Autodesk Inventor part; units mm, degrees
ref_plane "YZ Plane" through (0, 0, 0) normal (1, 0, 0) x (0, 1, 0)
ref_plane "XZ Plane" through (0, 0, 0) normal (0, 1, 0) x (-1, 0, 0)
ref_plane "XY Plane" through (0, 0, 0) normal (0, 0, 1) x (1, 0, 0)
sketch "Sketch1" plane through (0, 0, 0) normal (0, 1, 0) x (-1, 0, 0)
  circle A0 centre (0, 0) radius 41.275
  dimension "d0" = 82.55
extrude "Extrusion1" add sketch "Sketch1" along normal blind 0.75
sketch "Sketch2" plane through (0, 0.75, 0) normal (0, 1, 0) x (1, 0, 0)
  circle A0 centre (0, 0) radius 31.75
  circle A1 centre (0, 0) radius 41.275
  circle A2 centre (0, 0) radius 32.75
  circle A3 centre (0, 0) radius 40.275
  dimension "d3" = 63.5
  dimension "d4" = 1
  dimension "d5" = 1
extrude "Extrusion2" add sketch "Sketch2" along normal blind 12.7
fillet "Fillet1" radius 0.5 1 edges at (-32.75, 13.45, 0)
sketch "Sketch3" plane through (0, 0.75, 0) normal (0, 1, 0) x (1, 0, 0)
  circle A0 centre (0, 0) radius 17.4625 construction
  line L0 (0, 0) -> (0, -17.4625) construction
  circle A1 centre (0, -17.4625) radius 1.905
  circle A2 centre (15.123, -8.7313) radius 1.905
  circle A3 centre (15.123, 8.7312) radius 1.905
  circle A4 centre (0, 17.4625) radius 1.905
  circle A5 centre (-15.123, 8.7313) radius 1.905
  circle A6 centre (-15.123, -8.7312) radius 1.905
  dimension "d9" = 34.925
  dimension "d10" = 3.81
  dimension "d13" = 360
extrude "Extrusion3" cut sketch "Sketch3" against normal through all
thicken "Thicken1" operation cut thickness 6.35 both sides no extend neighbours no toward (0, -1, 0) faces at (-40.0621, 13.45, 7.3321)
properties part number "Mold - Wheel"
Here's how the part is built. I have some questions about the finished solid (model axes, mm). A direction names the side the tool comes from. Coordinates: 2 decimals unless noted, no trailing zeros. Write each loop counter-clockwise with the first axis right and the second up, starting at its lowest first coordinate (ties: lowest second). Pieces come first, ordered by that corner, then holes.
1) Which directions (+Z, -Z, +X, -X, +Y, -Y) give clear straight access to the entire face, cutting with the end or side of a thin tool? Please do faces 1 (the face through (-6.883, 7.011, -30.995)), 2 (the face through (-0.248, 0.38, 15.574)).
Filled in:
face 1: +Y
face 2: +Y, -Y
2) If we section it at C-C (y = 8.25): List the corners of the cut face in (x, z) for me.
Filled in:
outline: circle Ø65.5 at (0, 0); hole circle Ø63.5 at (0, 0)
3) If we section it at B-B (y = 1.75): List the corners of the cut face in (x, z) for me (3 decimals), plus the area to 3 significant figures.
Filled in:
outline: circle Ø82.55 at (0, 0); circle Ø65.5 at (0, 0); hole circle Ø80.55 at (0, 0); hole circle Ø63.5 at (0, 0)
area: 459 mm2
4) If I drill on line 1 (Z direction, x = 0, y = 7) (3 decimals); line 2 (X direction, y = 5, z = 19), over which ranges is the centre line in solid material (lowest first)?
Filled in:
line 1: z = -41.275 to -40.275, -32.75 to -31.75, 31.75 to 32.75, 40.275 to 41.275
line 2: x = -36.64 to -35.51, -26.68 to -25.44, 25.44 to 26.68, 35.51 to 36.64
5) I'm going to push flat-ended pins straight in: pin 1 (2 mm diameter, centred on y = 4, z = 14, fed in from +X); pin 2 (8 mm diameter, centred on x = -25, y = 8.5, fed in from -Z); pin 3 (3 mm diameter, centred on x = 24.5, y = 5.5, fed in from +Z). Where does each tip first touch, or does it pass through?
Filled in:
pin 1: stops at x = 39.17
pin 2: stops at z = -35.38
pin 3: stops at z = 34.27
